Could you check a few things on this drawing? It's one solid part, dimensions in mm from its lowest x, y, z. A direction names the side the tool comes from. Give positions to 0.01 mm unless a question says otherwise; leave off trailing zeros. Order: outer loops, then holes, each group sorted by start corner. A loop starts at its lowest first (then second) coordinate and runs counter-clockwise, first axis right, second up. Notation, with made-up numbers: (21, 48) -> (71, 48) arc R15 cw to (71, 55) -> close; hole circle Ø3 at (64.5, 35.5). An arc over 180 degrees is marked (long way). Answer as a JSON object with one key per item and string values.
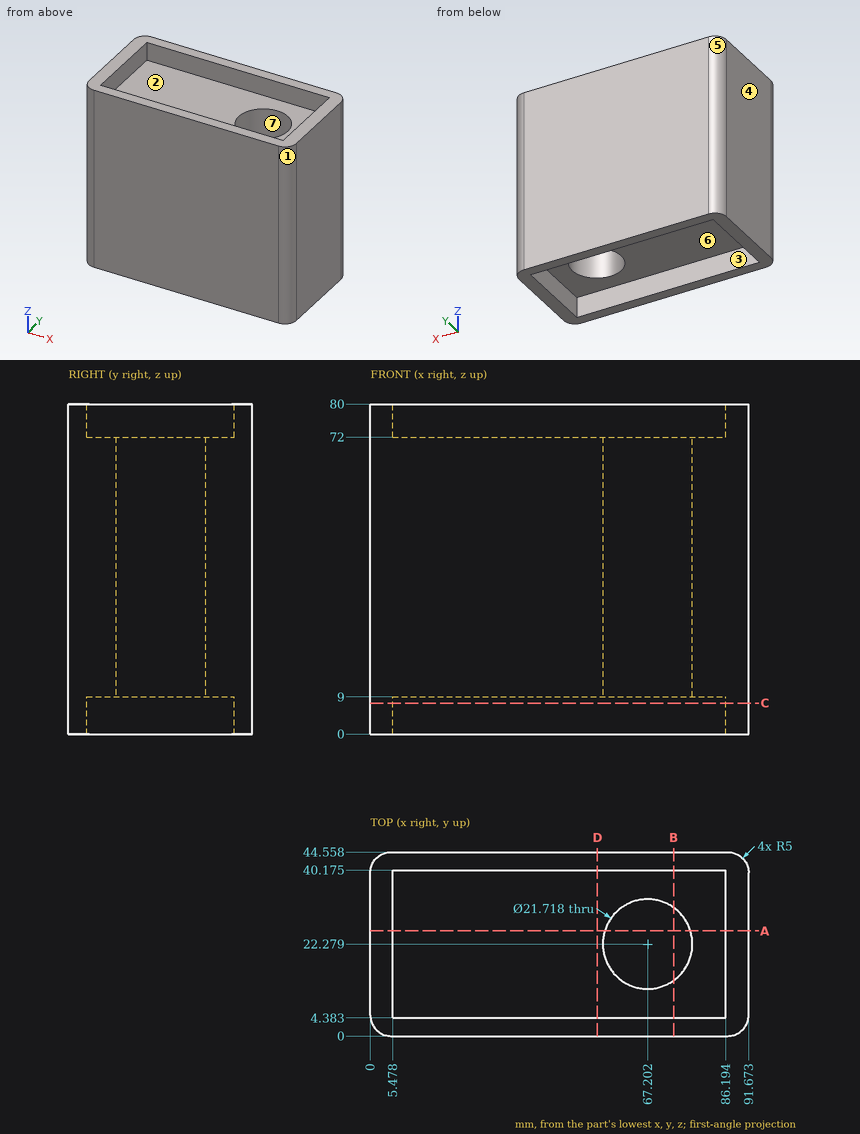
1. If we section it at D-D on x = 55: Please give me the cut outline in (y, z) (1 decimal).
Worked answers:
{"outline": "(0, 0) -> (4.4, 0) -> (4.4, 9) -> (40.2, 9) -> (40.2, 0) -> (44.6, 0) -> (44.6, 80) -> (40.2, 80) -> (40.2, 72) -> (4.4, 72) -> (4.4, 80) -> (0, 80) -> close"}
2. For the marked faces 1, 2 and 3, which set-ups out of +Z, -Z, +X, -X, +Y, -Y let a thin tool reach every point of the face, with its end or its side?
Worked answers:
{"face 1": "+Z, -Z, +X, -Y", "face 2": "+Z", "face 3": "-Z"}
3. If we mould it in two halves opening along Y, with no side actions, what happens to the marked faces 4, 5, 6 and 7? For each: +Y half, -Y half, draft (parallel to the pull), parting line (faces both ways), or undercut.
Worked answers:
{"face 4": "draft", "face 5": "+Y half", "face 6": "undercut", "face 7": "undercut"}
4. If we section it at C-C on z = 7.5: Please give me the cut outline in (x, y) (1 decimal).
Worked answers:
{"outline": "(0, 5) arc R5 ccw to (5, 0) -> (86.7, 0) arc R5 ccw to (91.7, 5) -> (91.7, 39.6) arc R5 ccw to (86.7, 44.6) -> (5, 44.6) arc R5 ccw to (0, 39.6) -> close; hole (5.5, 4.4) -> (86.2, 4.4) -> (86.2, 40.2) -> (5.5, 40.2) -> close"}
5. If we section it at A-A on y = 25.5: Please give me the cut outline in (x, z) (1 decimal), then the cut area to 4 significant figures.
Worked answers:
{"outline": "(0, 0) -> (5.5, 0) -> (5.5, 9) -> (56.8, 9) -> (56.8, 72) -> (5.5, 72) -> (5.5, 80) -> (0, 80) -> close; (77.6, 9) -> (86.2, 9) -> (86.2, 0) -> (91.7, 0) -> (91.7, 80) -> (86.2, 80) -> (86.2, 72) -> (77.6, 72) -> close", "area": "4,655 mm²"}
6. Please list where these lines run through material, in increasing order: L1, parallel to X at y = 6, z = 73 (1 decimal); L2, parallel to Y at x = 79, z = 75 (1 decimal); L3, parallel to Z at x = 45.5, y = 28.
Worked answers:
{"L1": "0 to 5.5, 86.2 to 91.7", "L2": "0 to 4.4, 40.2 to 44.6", "L3": "9 to 72"}
7. Will these pins go through, and if not, where does the flat tip stop? pin 1 Ø2 at (x, y) = (73.5, 36.5) entering from +Z; pin 2 Ø12 at (y, z) = (38, 60.5) entering from -X; pin 3 Ø8 at (x, y) = (69, 19.5) entering from +Z.
Worked answers:
{"pin 1": "z = 72", "pin 2": "x = 0", "pin 3": "through"}
8. If we section it at B-B on x = 73.5: Please give me the cut outline in (y, z) (1 decimal), then the cut area to 3 significant figures.
Worked answers:
{"outline": "(0, 0) -> (4.4, 0) -> (4.4, 9) -> (13.4, 9) -> (13.4, 72) -> (4.4, 72) -> (4.4, 80) -> (0, 80) -> close; (31.1, 9) -> (40.2, 9) -> (40.2, 0) -> (44.6, 0) -> (44.6, 80) -> (40.2, 80) -> (40.2, 72) -> (31.1, 72) -> close", "area": "1,840 mm²"}
